```python
from build123d import *

# Parameters (mm, degrees)
F0_R     = 5
F1_DEPTH = 45
F2_R     = 1
F3_DEPTH = 25
F4_SIZE  = 1


with BuildPart() as f1:
    # F0 (on Right) → F1 (new body)
    with BuildSketch(Plane.YZ):
        Circle(F0_R)
    extrude(amount=F1_DEPTH)

    # F2 (on face) → F3 (cut)
    with BuildSketch(Plane(origin=(0, 0, 0), x_dir=(0, -1, 0), z_dir=(-1, 0, 0))):
        Circle(F2_R)
    extrude(amount=-F3_DEPTH, mode=Mode.SUBTRACT)

    # F4
    f4_edges = [f1.edges().sort_by_distance(p)[0] for p in [
        (0, -5, 0),
        (45, -5, 0),
    ]]
    chamfer(f4_edges, length=F4_SIZE)


solid = f1.part
```
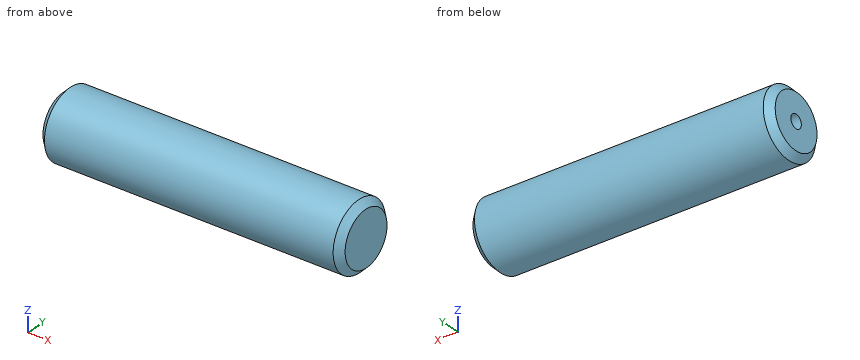
Build history of the part. All positions in model axes, mm. Round coordinates to 2 decimals unless told otherwise and drop trailing zeros. Order: outer loops, then holes, each group sorted by start corner. A loop starts at its lowest first (then second) coordinate and runs counter-clockwise, first axis right, second up. Notation, with made-up numbers: (64.25, 38.5) - (71.25, 38.5) arc R18 ccw to (71.25, 59.5) - close; hole circle Ø9 at (55.5, 19.25). An arc over 180 degrees is marked (long way). Use a Markdown table: item, result.
1) Saw through at C-C on x = 8. Write the cut outline in (y, z), and give its area (3 significant figures).
Recorded:
| item | result |
|---|---|
| outline | circle Ø10 at (0, 0); hole circle Ø2 at (0, 0) |
| area | 75.4 mm² |
2) Saw through at A-A on y = 0. Write the cut outline in (x, z).
Recorded:
| item | result |
|---|---|
| outline | (0, -4) - (1, -5) - (44, -5) - (45, -4) - (45, 4) - (44, 5) - (1, 5) - (0, 4) - (0, 1) - (25, 1) - (25, -1) - (0, -1) - close |
3) Flat gauge pins, fed straight in: pin 1 Ø3 at (x, z) = (15.5, 2.5) entering from +Y; pin 2 Ø1 at (x, z) = (25.5, 3) entering from +Y; pin 3 Ø3 at (x, y) = (33.5, -2) entering from +Z. Where does each tip first touch, or does it go through?
Recorded:
| item | result |
|---|---|
| pin 1 | stops at y = 4.9 |
| pin 2 | stops at y = 4.33 |
| pin 3 | stops at z = 4.97 |
4) Wall check: L1, parallel to Z at x = 18, y = 0; L2, parallel to Y at x = 14, z = -3; L3, parallel to Z at x = 2.5, y = -0.75. Give the ranges that are in metal, low to high.
Recorded:
| item | result |
|---|---|
| L1 | z = -5 to -1, 1 to 5 |
| L2 | y = -4 to 4 |
| L3 | z = -4.94 to -0.66, 0.66 to 4.94 |
5) Saw through at D-D on x = 30.5. Write the cut outline in (y, z).
Recorded:
| item | result |
|---|---|
| outline | circle Ø10 at (0, 0) |
